Model file for the job. Use its own axes, mm. A direction names the side the tool comes from. Round coordinates to 2 decimals unless told otherwise and drop trailing zeros. Order: outer loops, then holes, each group sorted by start corner. A loop starts at its lowest first (then second) coordinate and runs counter-clockwise, first axis right, second up. Notation, with made-up numbers: (46.5, 57) - (102.5, 57) arc R27 cw to (102.5, 91) - close; hole circle Ø10 at (45, 81). An arc over 180 degrees is marked (long way). Write item = value, one per line. Start each with the question number.
from build123d import *

# Parameters (mm, degrees)
SKETCH1_W           = 46.72
SKETCH1_H           = 65.06
SKETCH1_W_2         = 39.72
SKETCH1_H_2         = 53.61
BOSS_EXTRUDE1_DEPTH = 1.5
SKETCH1_3_W         = 46.72
SKETCH1_3_H         = 65.06
SKETCH1_3_W_2       = 43.72
SKETCH1_3_H_2       = 62.06
BOSS_EXTRUDE2_DEPTH = 30.24
SKETCH3_W           = 46.72
SKETCH3_H           = 65.06
SKETCH3_W_2         = 43.72
SKETCH3_H_2         = 62.06
SKETCH3_W_3         = 25.705
SKETCH3_H_3         = 50.55
BOSS_EXTRUDE3_DEPTH = 1.5
SKETCH4_R           = 10
SKETCH4_W           = 20
SKETCH4_H           = 5
CUT_EXTRUDE1_DEPTH  = 0.5


with BuildPart() as part:
    # Sketch1 → Boss-Extrude1 (new body)
    with BuildSketch(Plane.XY):
        with Locations((0, -2.475)):
            Rectangle(SKETCH1_W, SKETCH1_H)
        Rectangle(SKETCH1_W_2, SKETCH1_H_2, mode=Mode.SUBTRACT)
    extrude(amount=BOSS_EXTRUDE1_DEPTH)

    # Sketch1<3> → Boss-Extrude2 (add)
    with BuildSketch(Plane.XY):
        with Locations((0, -2.475)):
            Rectangle(SKETCH1_3_W, SKETCH1_3_H)
        with Locations((0, -2.475)):
            Rectangle(SKETCH1_3_W_2, SKETCH1_3_H_2, mode=Mode.SUBTRACT)
    extrude(amount=-BOSS_EXTRUDE2_DEPTH)

    # Sketch3 → Boss-Extrude3 (add)
    # profile 1 of 2: a face of its own
    with BuildSketch(Plane(origin=(0, 0, -30.24), x_dir=(-1, 0, 0), z_dir=(0, 0, -1))):
        with Locations((0, -2.475)):
            Rectangle(SKETCH3_W, SKETCH3_H)
        with Locations((0, -2.475)):
            Rectangle(SKETCH3_W_2, SKETCH3_H_2, mode=Mode.SUBTRACT)
    # profile 2 of 2: a face of its own
    with BuildSketch(Plane(origin=(0, 0, -30.24), x_dir=(-1, 0, 0), z_dir=(0, 0, -1))):
        with Locations((0, -2.475)):
            Rectangle(SKETCH3_W_2, SKETCH3_H_2)
        with Locations((-6.7605, 1.08)):
            Rectangle(SKETCH3_W_3, SKETCH3_H_3, mode=Mode.SUBTRACT)
    extrude(amount=BOSS_EXTRUDE3_DEPTH)

    # Sketch4 → Cut-Extrude1 (cut)
    with BuildSketch(Plane(origin=(23.36, 0, 0), x_dir=(0, 0, -1), z_dir=(1, 0, 0))):
        with Locations(Location((16.3, 16.055, 0), (0, 0, 90))):
            Circle(SKETCH4_R)
        with Locations((16.3, -21.945)):
            Rectangle(SKETCH4_W, SKETCH4_H)
    extrude(amount=-CUT_EXTRUDE1_DEPTH, mode=Mode.SUBTRACT)


solid = part.part
Item 1: Saw through at B-B, the plane z = -16.3. Give the cut face in (x, y) (3 decimals).
Item 2: Probe L1, parallel to X at y = -12, z = -9.5; L2, parallel to Y at x = -10, z = -20.5 (3 decimals); L3, parallel to Z at x = -15.5, y = -0.5. List the from-to ranges inside material, lowest first.
Item 3: Saw through at D-D, the plane x = -18. Give the cut face in (y, z) (3 decimals), then the cut area to 3 significant figures.
Item 4: Mould opens along Y. For faces 6 (the face through (23.114, 25.593, -13.296)), 7 (the face through (-10, -2, -31.74)), 8 (the face through (0, -35.005, -15)) say: +Y half, -Y half, draft (parallel to the pull), parting line (faces both ways), or undercut.
Item 5: Saw through at A-A, the plane x = 10. Give the cut face in (y, z) (3 decimals), then the cut area to 3 significant figures.
Item 6: Which spindle directions (+Z, -Z, +X, -X, +Y, -Y) get a long thin tool onto all of the face, cutting with end or side? Do faces 1 (the face through (20.4, -2, 1.5)), 2 (the face through (22.86, -22, -16)), 3 (the face through (0, -28, 0)), 4 (the face through (19.86, 0, 1)), 5 (the face through (7, 26.355, -31)). Say none if no direction does.
Item 7: Drop flat-ended pins along their axis: pin 1 (3 mm diameter, centred on x = -8, y = -6.5, fed in from +Z); pin 2 (2.5 mm diameter, centred on y = -22.5, z = -18, fed in from +X). Give the stop position or say it passes through.
Item 8: Saw through at C-C, the plane y = -11. Give the cut face in (x, z).
Check sheet entries:
q1.outline = (-23.36, -35.005) - (23.36, -35.005) - (23.36, -24.445) - (22.86, -24.445) - (22.86, -19.445) - (23.36, -19.445) - (23.36, 6.055) - (22.86, 6.055) - (22.86, 26.055) - (23.36, 26.055) - (23.36, 30.055) - (-23.36, 30.055) - close; hole (-21.86, -33.505) - (21.86, -33.505) - (21.86, 28.555) - (-21.86, 28.555) - close
q2.L1 = -23.36 to -21.86, 21.86 to 23.36
q2.L2 = -35.005 to -33.505, 28.555 to 30.055
q2.L3 = -31.74 to -30.24
q3.outline = (-35.005, -31.74) - (30.055, -31.74) - (30.055, 1.5) - (26.805, 1.5) - (26.805, 0) - (28.555, 0) - (28.555, -30.24) - (-33.505, -30.24) - (-33.505, 0) - (-26.805, 0) - (-26.805, 1.5) - (-35.005, 1.5) - close
q3.area = 205 mm2
q4.face_6 = undercut
q4.face_7 = draft
q4.face_8 = -Y half
q5.outline = (-35.005, -31.74) - (-24.195, -31.74) - (-24.195, -30.24) - (-33.505, -30.24) - (-33.505, 0) - (-26.805, 0) - (-26.805, 1.5) - (-35.005, 1.5) - close; (26.355, -31.74) - (30.055, -31.74) - (30.055, 1.5) - (26.805, 1.5) - (26.805, 0) - (28.555, 0) - (28.555, -30.24) - (26.355, -30.24) - close
q5.area = 130 mm2
q6.face_1 = +Z, +X, -X, +Y, -Y
q6.face_2 = +X
q6.face_3 = none
q6.face_4 = +Z
q6.face_5 = +Z, -Z
q7.pin_1 = -30.24
q7.pin_2 = 22.86
q8.outline = (-23.36, -31.74) - (-6.09, -31.74) - (-6.09, -30.24) - (-21.86, -30.24) - (-21.86, 0) - (-19.86, 0) - (-19.86, 1.5) - (-23.36, 1.5) - close; (19.61, -31.74) - (23.36, -31.74) - (23.36, 1.5) - (19.86, 1.5) - (19.86, 0) - (21.86, 0) - (21.86, -30.24) - (19.61, -30.24) - close
